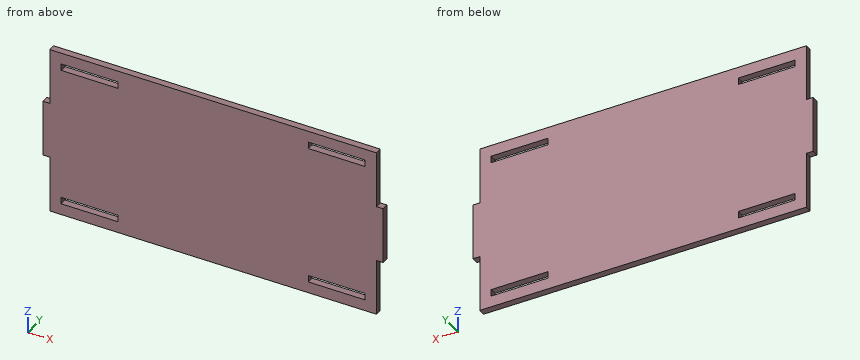
Autodesk Inventor part; units mm, degrees
ref_plane "YZ Plane" through (0, 0, 0) normal (1, 0, 0) x (0, 1, 0)
ref_plane "XZ Plane" through (0, 0, 0) normal (0, 1, 0) x (-1, 0, 0)
ref_plane "XY Plane" through (0, 0, 0) normal (0, 0, 1) x (1, 0, 0)
sketch "Sketch1" plane through (0, 0, 0) normal (0, 1, 0) x (-1, 0, 0)
  line L0 (71.1097, -38.0648) -> (71.1097, -13.0648)
  line L1 (71.1097, -13.0648) -> (74.1097, -13.0648)
  line L2 (74.1097, -13.0648) -> (74.1097, 11.9352)
  line L3 (74.1097, 11.9352) -> (71.1097, 11.9352)
  line L4 (71.1097, 11.9352) -> (71.1097, 36.9352)
  line L5 (-72.8903, -38.0648) -> (-72.8903, -13.0648)
  line L6 (-72.8903, 36.9352) -> (-72.8903, 11.9352)
  line L7 (-72.8903, -13.0648) -> (-75.8903, -13.0648)
  line L8 (-75.8903, -13.0648) -> (-75.8903, 11.9352)
  line L9 (-75.8903, 11.9352) -> (-72.8903, 11.9352)
  line L10 (71.1097, -38.0648) -> (-72.8903, -38.0648)
  line L11 (71.1097, 36.9352) -> (-72.8903, 36.9352)
  point P0 (0, 0)
extrude "Extrusion1" add sketch "Sketch1" along normal blind 3
sketch "Sketch2" plane through (0, 3, 0) normal (0, 1, 0) x (1, 0, 0)
  line L0 (-71.1097, -36.9352) -> (72.8903, -36.9352)
  line L1 (-66.1097, -31.9352) -> (-56.1097, -31.9352)
  line L2 (-56.1097, -31.9352) -> (-56.1097, -28.9352)
  line L3 (-56.1097, -28.9352) -> (-66.1097, -28.9352)
  line L4 (-66.1097, -28.9352) -> (-66.1097, -31.9352)
  line L5 (72.8903, 38.0648) -> (-71.1097, 38.0648)
  line L6 (-56.1097, 30.0648) -> (-66.1097, 30.0648)
  line L7 (-66.1097, 30.0648) -> (-66.1097, 33.0648)
  line L8 (-66.1097, 33.0648) -> (-56.1097, 33.0648)
  line L9 (-56.1097, 33.0648) -> (-56.1097, 30.0648)
  line L10 (67.8903, 33.0648) -> (57.8903, 33.0648)
  line L11 (57.8903, 33.0648) -> (57.8903, 30.0648)
  line L12 (57.8903, 30.0648) -> (67.8903, 30.0648)
  line L13 (67.8903, 30.0648) -> (67.8903, 33.0648)
  line L14 (67.8903, -31.9352) -> (57.8903, -31.9352)
  line L15 (57.8903, -31.9352) -> (57.8903, -28.9352)
  line L16 (57.8903, -28.9352) -> (67.8903, -28.9352)
  line L17 (67.8903, -28.9352) -> (67.8903, -31.9352)
  point P0 (0, 0)
extrude "Extrusion2" cut sketch "Sketch2" against normal blind 30
sketch "Sketch3" plane through (0, 3, 0) normal (0, 1, 0) x (1, 0, 0)
  line L0 (72.8903, 38.0648) -> (-71.1097, 38.0648)
  circle A0 centre (-14.1097, 28.0648) radius 5
  circle A1 centre (15.8903, 28.0648) radius 5
  line L1 (-71.1097, -36.9352) -> (72.8903, -36.9352)
  circle A2 centre (-14.1097, -26.9352) radius 5
  circle A3 centre (15.8903, -26.9352) radius 5
  point P0 (0, 0)
  dimension "d35" = 10
  dimension "d36" = 10
  dimension "d39" = 10
  dimension "d40" = 10
extrude "Extrusion3" cut sketch "Sketch3" against normal blind 30
sketch "Sketch4" plane through (0, 3, 0) normal (0, 1, 0) x (1, 0, 0)
  line L0 (-56.1097, 33.0648) -> (-56.1097, 30.0648)
  line L1 (-56.1097, 33.0648) -> (-41.1097, 33.0648)
  line L2 (-41.1097, 33.0648) -> (-41.1097, 30.0648)
  line L3 (-41.1097, 30.0648) -> (-56.1097, 30.0648)
  line L4 (-56.1097, 30.0648) -> (-56.1097, 33.0648)
  line L5 (57.8903, 33.0648) -> (42.8903, 33.0648)
  line L6 (42.8903, 33.0648) -> (42.8903, 30.0648)
  line L7 (42.8903, 30.0648) -> (57.8903, 30.0648)
  line L8 (57.8903, 30.0648) -> (57.8903, 33.0648)
  line L9 (-56.1097, -31.9352) -> (-66.1097, -31.9352)
  line L10 (-56.1097, -31.9352) -> (-41.1097, -31.9352)
  line L11 (-41.1097, -31.9352) -> (-41.1097, -28.9352)
  line L12 (-41.1097, -28.9352) -> (-56.1097, -28.9352)
  line L13 (-56.1097, -28.9352) -> (-56.1097, -31.9352)
  line L14 (57.8903, -31.9352) -> (57.8903, -28.9352)
  line L15 (57.8903, -31.9352) -> (42.8903, -31.9352)
  line L16 (42.8903, -31.9352) -> (42.8903, -28.9352)
  line L17 (42.8903, -28.9352) -> (57.8903, -28.9352)
  line L18 (57.8903, -28.9352) -> (57.8903, -31.9352)
  point P0 (0, 0)
  dimension "d43" = 15
  dimension "d44" = 15
extrude "Extrusion4" cut sketch "Sketch4" against normal blind 10
sketch "Sketch5" plane through (0, 3, 0) normal (0, 1, 0) x (1, 0, 0)
  circle A0 centre (-14.1097, 28.0648) radius 5
  circle A1 centre (-14.1097, 28.0648) radius 5
  circle A2 centre (15.8903, 28.0648) radius 5
  circle A3 centre (15.8903, 28.0648) radius 5
  circle A4 centre (15.8903, -26.9352) radius 5
  circle A5 centre (15.8903, -26.9352) radius 5
  circle A6 centre (-14.1097, -26.9352) radius 5
  circle A7 centre (-14.1097, -26.9352) radius 5
  point P0 (0, 0)
extrude "Extrusion5" add sketch "Sketch5" against normal blind 3
properties part number "Level1 (Motoren)"
Geometry: final body of the model. Coordinates: model frame, mm. Coordinates: 2 decimals unless noted, no trailing zeros. Order: outer loops, then holes, each group sorted by start corner. A loop starts at its lowest first (then second) coordinate and runs counter-clockwise, first axis right, second up. Notation, with made-up numbers: (-11.5, -4.5) - (45.5, -4.5) arc R19 ccw to (45.5, 5.5) - close; hole circle Ø11 at (40.5, 48). An arc over 180 degrees is marked (long way). Write each question's results on one line, items separated by ' | '.
1) Section B-B, the plane x = -57.5. Return loops of the section in (y, z).
Results list:
outline: (0, -38.06) - (3, -38.06) - (3, -33.06) - (0, -33.06) - close; (0, -30.06) - (3, -30.06) - (3, 28.94) - (0, 28.94) - close; (0, 31.94) - (3, 31.94) - (3, 36.94) - (0, 36.94) - close
2) Line query: line 1 (X direction, y = 2.2, z = 29); line 2 (Z direction, x = -65, y = 2.65); line 3 (X direction, y = 2, z = -21). Output: solid intervals per line, ascending. Write a range as from..to.
Results list:
line 1: -71.11..-66.11, -41.11..42.89, 67.89..72.89 | line 2: -38.06..-33.06, -30.06..28.94, 31.94..36.94 | line 3: -71.11..72.89
3) Section C-C, the plane z = -15.5. Return loops of the section in (x, y), plus the area to 3 significant figures.
Results list:
outline: (-71.11, 0) - (72.89, 0) - (72.89, 3) - (-71.11, 3) - close | area: 432 mm^2
4) Pin query (flat end, axial travel): pin 1 (0.9 mm diameter, centred on y = 2, z = -25.5, fed in from -X); pin 2 (1.5 mm diameter, centred on y = 0.5, z = -24, fed in from +X); pin 3 (1.5 mm diameter, centred on x = -72.5, y = 1, fed in from -Z). Return the tip coordinate at first contact, or that it passes through.
Results list:
pin 1: x = -71.11 | pin 2: x = 72.89 | pin 3: z = -13.06
5) Section A-A, the plane y = 2.4. Return loops of the section in (x, z).
Results list:
outline: (-74.11, -13.06) - (-71.11, -13.06) - (-71.11, -38.06) - (72.89, -38.06) - (72.89, -13.06) - (75.89, -13.06) - (75.89, 11.94) - (72.89, 11.94) - (72.89, 36.94) - (-71.11, 36.94) - (-71.11, 11.94) - (-74.11, 11.94) - close; hole (-66.11, -33.06) - (-41.11, -33.06) - (-41.11, -30.06) - (-66.11, -30.06) - close; hole (-66.11, 28.94) - (-41.11, 28.94) - (-41.11, 31.94) - (-66.11, 31.94) - close; hole (42.89, -33.06) - (67.89, -33.06) - (67.89, -30.06) - (42.89, -30.06) - close; hole (42.89, 28.94) - (67.89, 28.94) - (67.89, 31.94) - (42.89, 31.94) - close
